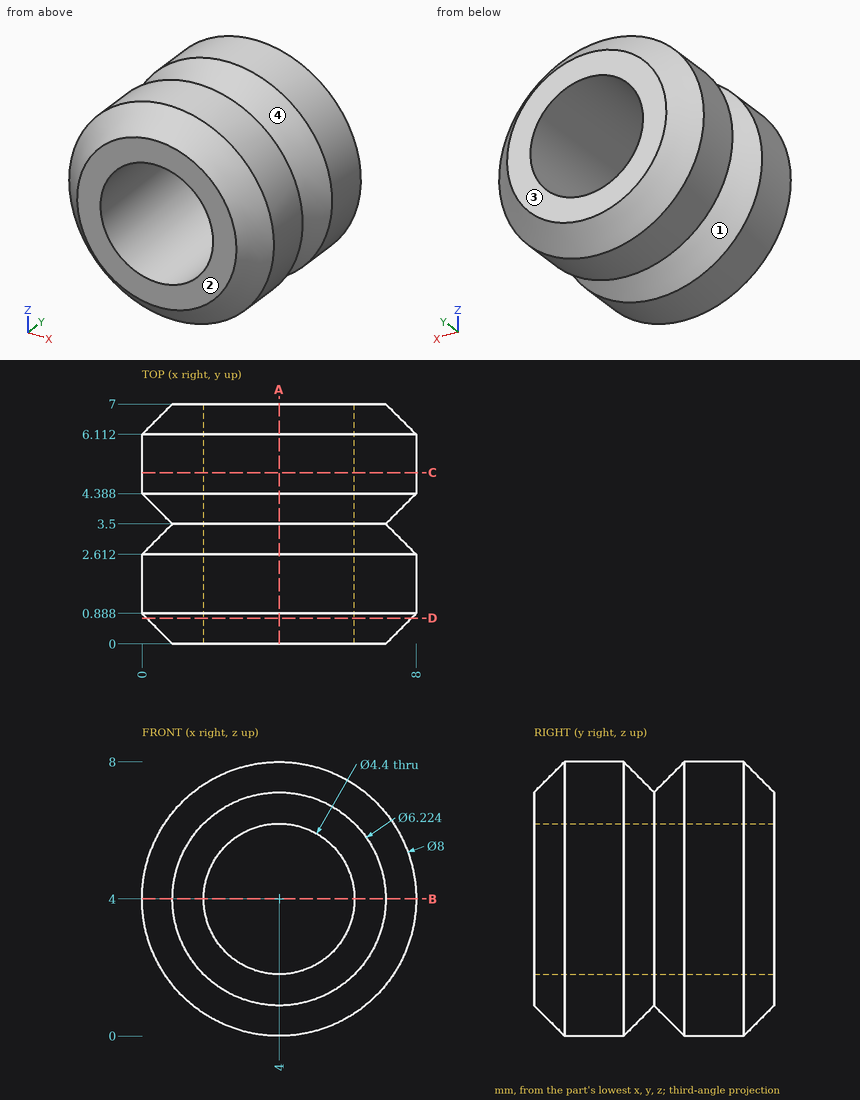
Design review of the part shown in the three views and the two pictorial views. Dimensions are in mm from the part's minimum x, y and z. Coordinates: 2 decimals unless noted, no trailing zeros. Order: outer loops, then holes, each group sorted by start corner. A loop starts at its lowest first (then second) coordinate and runs counter-clockwise, first axis right, second up. Notation, with made-up numbers: (55.5, 29) -> (107.5, 29) arc R6 ccw to (107.5, 40) -> close; hole circle Ø5 at (27.25, 40). An arc over 180 degrees is marked (long way). Use one line per item in the form item = value. Start each with the question number.
(1) Add section D-D on y = 0.75. State the section outline as (x, z) points.
(2) Insertion check: pin 1 (2 mm diameter, centred on x = 2.5, y = 2.5, fed in from +Z); pin 2 (2 mm diameter, centred on x = 5.5, z = 5.5, fed in from +Y); pin 3 (1 mm diameter, centred on y = 5, z = 2.5, fed in from -X); pin 4 (2 mm diameter, centred on y = 0.5, z = 1, fed in from +X). Each pin has a flat end and moves straight along its axis. Give the tip position at first contact, or say it passes through.
(3) Add section A-A on x = 4. State the section outline as (y, z) points.
(4) For probe 1 along Z at (x, y) = (4, 2); probe 2 along Y at (x, z) = (0.5, 3), list the stretches that pass through material, from the lowest coordinate up.
(5) The part is to be moulded in two halves that separate along Y. For the marked faces 1, 2, 3 and 4, say which applies: +Y half, -Y half, draft (parallel to the pull), parting line (faces both ways), or undercut.
(6) Add section B-B on z = 4. State the section outline as (x, y) points.
(7) Add section C-C on y = 5. State the section outline as (x, z) points.
Answer block:
q1.outline = circle Ø7.72 at (4, 4); hole circle Ø4.4 at (4, 4)
q2.pin_1 = 7.97
q2.pin_2 = 7
q2.pin_3 = 0.13
q2.pin_4 = 7.42
q3.outline = (0, 0.89) -> (0.89, 0) -> (2.61, 0) -> (3.5, 0.89) -> (4.39, 0) -> (6.11, 0) -> (7, 0.89) -> (7, 1.8) -> (0, 1.8) -> close; (0, 6.2) -> (7, 6.2) -> (7, 7.11) -> (6.11, 8) -> (4.39, 8) -> (3.5, 7.11) -> (2.61, 8) -> (0.89, 8) -> (0, 7.11) -> close
q4.probe_1 = 0 to 1.8, 6.2 to 8
q4.probe_2 = 0.53 to 2.97, 4.03 to 6.47
q5.face_1 = undercut
q5.face_2 = -Y half
q5.face_3 = +Y half
q5.face_4 = undercut
q6.outline = (0, 0.89) -> (0.89, 0) -> (1.8, 0) -> (1.8, 7) -> (0.89, 7) -> (0, 6.11) -> (0, 4.39) -> (0.89, 3.5) -> (0, 2.61) -> close; (6.2, 0) -> (7.11, 0) -> (8, 0.89) -> (8, 2.61) -> (7.11, 3.5) -> (8, 4.39) -> (8, 6.11) -> (7.11, 7) -> (6.2, 7) -> close
q7.outline = circle Ø8 at (4, 4); hole circle Ø4.4 at (4, 4)
